Autodesk Fusion 360 part; units mm, degrees
sketch "Sketch1" plane through (0, 0, 0) normal (1, 0, 0) x (0, 0, -1)
  circle A0 centre (0, 0) radius 2.3995
  dimension "d1" = 4.799
extrude "Extrude1" add sketch "Sketch1" along normal blind 36
sketch "Sketch2" plane through (36, 0, 0) normal (1, 0, 0) x (0, 0, -1)
  circle A0 centre (0, 0) radius 2.3995
  line L0 (0.7, 2.3995) -> (-0.7, 2.3995)
  line L1 (-0.7, -2.3995) -> (0.7, -2.3995)
  line L2 (0.7, 2.3995) -> (-0.7, -2.3995) construction
  line L3 (-0.7, 2.3995) -> (0.7, -2.3995) construction
  line L4 (-2.3995, 0.7) -> (-2.3995, -0.7)
  line L5 (2.3995, -0.7) -> (2.3995, 0.7)
  line L6 (2.3995, 0.7) -> (-2.3995, -0.7) construction
  line L7 (-2.3995, 0.7) -> (2.3995, -0.7) construction
  line L8 (-0.7, 2.3995) -> (-0.7, 1)
  line L9 (-0.7, -1) -> (-0.7, -2.3995)
  line L10 (-2.3995, -0.7) -> (-1, -0.7)
  line L11 (1, -0.7) -> (2.3995, -0.7)
  line L12 (0.7, -2.3995) -> (0.7, -1)
  line L13 (0.7, 1) -> (0.7, 2.3995)
  line L14 (2.3995, 0.7) -> (1, 0.7)
  line L15 (-1, 0.7) -> (-2.3995, 0.7)
  arc A1 (-1, 0.7) -> (-0.7, 1) centre (-1, 1) ccw
  arc A2 (0.7, 1) -> (1, 0.7) centre (1, 1) ccw
  arc A3 (1, -0.7) -> (0.7, -1) centre (1, -1) ccw
  arc A4 (-0.7, -1) -> (-1, -0.7) centre (-1, -1) ccw
  dimension "d4" = 4.799
  dimension "d5" = 1.4
  dimension "d6" = 4.799
  dimension "d7" = 1.4
  dimension "d8" = 0.3
  dimension "d11" = 0.3
extrude "Extrude2" cut sketch "Sketch2" against normal blind 27 contours A0 L13 L14 A2 | A0 L11 L12 A3 | A0 L8 L15 A1 | A0 L9 L10 A4
sketch "Sketch4" plane through (0, 0, 0) normal (-1, 0, 0) x (0, 0, 1)
  circle A0 centre (0, 0) radius 2.3995
  circle A1 centre (0, 0) radius 2.3995
  arc A2 (2.2951, 0.7) -> (0.7, 2.2951) centre (0, 0) ccw
extrude "Extrude4" cut sketch "Sketch4" against normal blind 9
sketch "Sketch5" plane through (9, 0, 0) normal (-1, 0, 0) x (0, 0, 1)
  line L0 (-2.2951, -0.7) -> (-1, -0.7)
  arc A0 (-0.7, -1) -> (-1, -0.7) centre (-1, -1) ccw
  line L1 (-0.7, -1) -> (-0.7, -2.2951)
  arc A1 (-0.7, -2.2951) -> (0.7, -2.2951) centre (0, 0) ccw
  line L2 (0.7, -2.2951) -> (0.7, -1)
  arc A2 (1, -0.7) -> (0.7, -1) centre (1, -1) ccw
  line L3 (1, -0.7) -> (2.2951, -0.7)
  arc A3 (2.2951, -0.7) -> (2.2951, 0.7) centre (0, 0) ccw
  line L4 (2.2951, 0.7) -> (1, 0.7)
  arc A4 (0.7, 1) -> (1, 0.7) centre (1, 1) ccw
  line L5 (0.7, 1) -> (0.7, 2.2951)
  arc A5 (0.7, 2.2951) -> (-0.7, 2.2951) centre (0, 0) ccw
  line L6 (-0.7, 2.2951) -> (-0.7, 1)
  arc A6 (-1, 0.7) -> (-0.7, 1) centre (-1, 1) ccw
  line L7 (-1, 0.7) -> (-2.2951, 0.7)
  arc A7 (-2.2951, 0.7) -> (-2.2951, -0.7) centre (0, 0) ccw
  circle A8 centre (0, 0) radius 3
  dimension "d19" = 6
extrude "Extrude5" add sketch "Sketch5" along normal blind 5 contours L0 A0 L1 A1 L2 A2 L3 A3 L4 A4 L5 A5 L6 A6 L7 A7 | A8
sketch "Sketch6" plane through (4, 0, 0) normal (-1, 0, 0) x (0, 0, 1)
  circle A0 centre (0, 0) radius 3
  line L0 (-1.25, 0) -> (-1.25, 1.3297)
  line L1 (-2.2951, 0.7) -> (-1, 0.7)
  line L2 (-1.25, 1.3297) -> (-1.25, -1.3297)
  arc A1 (-1.25, -1.3297) -> (-1.25, 1.3297) centre (0, 0) ccw
  point P0 (-0.7, -2.2951)
  dimension "d22" = 3.65
  dimension "d23" = 1.25
extrude "Extrude6" cut sketch "Sketch6" against normal blind 9 contours L0 L2 A1
fillet "Fillet3" radius 0.5 16 edges at (36, 2.3995, 0) (36, 0.7, -1.6476) (36, 0.7879, -0.7879) (36, 1.6476, -0.7) (36, 1.6476, 0.7) (36, 0.7879, 0.7879) (36, 0.7, 1.6476) (36, 0, 2.3995) (36, -0.7, 1.6476) (36, -0.7879, 0.7879) (36, -1.6476, 0.7) (36, -2.3995, 0) (36, -1.6476, -0.7) (36, -0.7879, -0.7879) (36, -0.7, -1.6476) (36, 0, -2.3995)
Here's how the part is built. I have some questions about the finished solid (model axes, mm). A direction names the side the tool comes from. Coordinates: 2 decimals unless noted, no trailing zeros. Loops run counter-clockwise (first coordinate to the right, second up) from the corner with the lowest first, then second, coordinate; pieces in that order, holes last. Notation, with made-up numbers: (9.5, 80) -> (38.5, 80) arc R26 cw to (38.5, 94) -> close; hole circle Ø5 at (22.25, 66.25). An arc over 180 degrees is marked (long way). Return JSON: item names as keys, results as strings.
1) Will these pins go through, and if not, where does the flat tip stop? pin 1 (1 mm diameter, centred on x = 18.5, y = 0, fed in from -Z); pin 2 (3 mm diameter, centred on x = 11.5, z = -1, fed in from -Y); pin 3 (0.6 mm diameter, centred on x = 18.5, z = -2, fed in from +Y).
Results below:
{"pin 1": "z = -2.4", "pin 2": "y = -2.4", "pin 3": "y = 0.7"}
2) If we section it at B-B, the plane z = -1.6: Write out the boundary of the cut face in (x, y).
Results below:
{"outline": "(4, -2.54) -> (9, -2.54) -> (9, -0.7) -> (35.5, -0.7) arc R0.5 ccw to (36, -0.2) -> (36, 0.2) arc R0.5 ccw to (35.5, 0.7) -> (9, 0.7) -> (9, 2.54) -> (4, 2.54) -> close"}
3) Thinking about a two-plate mould opening in Z: for faces 1 (the face through (7.437, -0.059, 1.824)), 2 (the face through (22, 2, -0.7)), 3 (the face through (22, -2, 0.7)), 4 (the face through (7, 0, -1.25)), which applies, +Z half, -Z half, draft (parallel to the pull), parting line (faces both ways), or undercut?
Results below:
{"face 1": "undercut", "face 2": "-Z half", "face 3": "+Z half", "face 4": "undercut"}
4) If we section it at A-A, the plane x = 29: Write out the boundary of the cut face in (y, z).
Results below:
{"outline": "(-2.3, -0.7) -> (-1, -0.7) arc R0.3 cw to (-0.7, -1) -> (-0.7, -2.3) arc R2.4 ccw to (0.7, -2.3) -> (0.7, -1) arc R0.3 cw to (1, -0.7) -> (2.3, -0.7) arc R2.4 ccw to (2.3, 0.7) -> (1, 0.7) arc R0.3 cw to (0.7, 1) -> (0.7, 2.3) arc R2.4 ccw to (-0.7, 2.3) -> (-0.7, 1) arc R0.3 cw to (-1, 0.7) -> (-2.3, 0.7) arc R2.4 ccw to start"}
5) For faces 5 (the face through (22, -2, -0.7)), 6 (the face through (13, 0, 0)), 7 (the face through (22.1, 0, 2.4)), which set-ups out of +Z, -Z, +X, -X, +Y, -Y let a thin tool reach every point of the face, with its end or its side?
Results below:
{"face 5": "-Z, +X, -Y", "face 6": "-X", "face 7": "+Z, +X"}
6) I need wall thicknesses on line 1 (Y direction, x = 10.75, z = 0) (1 decimal); line 2 (Y direction, x = 8.75, z = 0) (3 decimals); line 3 (X direction, y = 1.35, z = 1.45). Which ranges of each line are inside material? Lowest first, please. Write a range as from..to.
Results below:
{"line 1": "-2.4..-1.8, 1.8..2.4", "line 2": "-3..-1.825, 1.825..3", "line 3": "4..9"}
